The listing builds one solid part. Answer for the finished solid, in the listing's coordinates (mm). A direction names the side the tool comes from. Coordinates: 2 decimals unless noted, no trailing zeros. Order: outer loops, then holes, each group sorted by start corner. A loop starts at its lowest first (then second) coordinate and runs counter-clockwise, first axis right, second up. Notation, with made-up numbers: M -28,-18 L 13,-18 A16 cw 13,-13 Z; hole C 70.5,88.25 d7. An arc over 180 degrees is marked long. One line per item, written item: value. Start each with the question number.
Q1. The part is cut by section B-B on y = -15. Give the vertices of the cut face in (x, z) (3 decimals).
Q2. Each of these flat-tipped pins is pushed along its axis until it touches: pin 1 Ø1 at (y, z) = (-14.5, 1) entering from -X; pin 2 Ø1 at (x, z) = (33, 2) entering from -Y (3 decimals). Where does it stop, or does it pass through?
Q3. Straight lines are drawn through the part: line 1 along X through (y, z) = (-2, 2.35); line 2 along X through (y, z) = (5, 0.35); line 3 along X through (y, z) = (13, 2.4). For each, find the intervals that lie inside material, in ascending order. Write a range as [from, to].
Q4. For faces 1 (the flat face through (-31.75, 0, 2)), 2 (the flat face through (31.75, 0, 2)), 3 (the flat face through (33, -10.795, 2)), 4 (the flat face through (33, 10.795, 2)), 5 (the flat face through (-31.75, 14, 2)), determine the directions among +Z, -Z, +X, -X, +Y, -Y from which every point of the face is accessible in a straight line to the end or side of a thin tool.
Q5. The part is cut by section A-A on z = 1.65. Give the number of separate pieces and of enclosed holes in the cut face, then the cut area to 3 significant figures.
Q6. Determine the mould class of faces 6 (the flat face through (0, 0, 0)), 7 (the flat face through (-33, -10.795, 2)), 8 (the flat face through (33, 4.445, 2)) for opening direction Y: pulls with the +Y half, pulls with the -Y half, needs draft (parallel to the pull), parting line crosses it, or undercut.
```python
from build123d import *

# Parameters (mm, degrees)
SKETCH1_W                      = 63.5
SKETCH1_H                      = 34.29
BOSS_EXTRUDE1_DEPTH            = 3.175
SKETCH2_W                      = 3.2258
SKETCH2_H                      = 6.35
BOSS_EXTRUDE2_DEPTH            = 3.175
SKETCH3_RX                     = 10.16
SKETCH3_RY                     = 6.35
CUT_FOR_LIP_MOTOR_CABLES_DEPTH = 4.175


with BuildPart() as part:
    # Sketch1 → Boss-Extrude1 (new body)
    with BuildSketch(Plane.XY):
        Rectangle(SKETCH1_W, SKETCH1_H)
    extrude(amount=BOSS_EXTRUDE1_DEPTH)

    # Sketch2 → Boss-Extrude2 (add)
    with BuildSketch(Plane.XY.offset(3.175)):
        with Locations((-33.3629, 7.62)):
            Rectangle(SKETCH2_W, SKETCH2_H)
        with Locations((-33.3629, -7.62)):
            Rectangle(SKETCH2_W, SKETCH2_H)
    boss_extrude2 = extrude(amount=-BOSS_EXTRUDE2_DEPTH)

    # Mirror1: Boss-Extrude2 across plane
    add(boss_extrude2.mirror(Plane(origin=(0, 0, 0), x_dir=(0, 0, 1), z_dir=(1, 0, 0))))

    # Sketch3 → cut for lip motor cables (cut, through all)
    with BuildSketch(Plane(origin=(0, 0, 0), x_dir=(-1, 0, 0), z_dir=(0, 0, -1))):
        with Locations(Location((-14.992180724, 0), (0, 0, 180))):
            Ellipse(SKETCH3_RX, SKETCH3_RY)
    cut_for_lip_motor_cables = extrude(amount=-CUT_FOR_LIP_MOTOR_CABLES_DEPTH, mode=Mode.SUBTRACT)

    # Mirror2: cut for lip motor cables across plane
    add(cut_for_lip_motor_cables.mirror(Plane(origin=(0, 0, 0), x_dir=(0, 0, 1), z_dir=(1, 0, 0))), mode=Mode.SUBTRACT)


solid = part.part
```
Output:
1. outline: M -31.75,0 L 31.75,0 L 31.75,3.175 L -31.75,3.175 Z
2. pin 1: stops at x = -31.75
2. pin 2: stops at y = -10.795
3. line 1: x = [-31.75, -24.64], [-5.35, 5.35], [24.64, 31.75]
3. line 2: x = [-34.98, -21.26], [-8.73, 8.73], [21.26, 34.98]
3. line 3: x = [-31.75, 31.75]
4. face 1: +Z, -Z, -X
4. face 2: +Z, -Z, +X
4. face 3: +Z, -Z, +X, -Y
4. face 4: +Z, -Z, +X, +Y
4. face 5: +Z, -Z, -X, +Y
5. separate pieces: 1
5. enclosed holes: 2
5. area: 1,850 mm^2
6. face 6: needs draft
6. face 7: pulls with the -Y half
6. face 8: undercut
